Check sheet for the modelled part. Datum: model origin and axes. Units: mm. A direction names the side the tool comes from. Coordinates: 2 decimals unless noted, no trailing zeros. Loops run counter-clockwise (first coordinate to the right, second up) from the corner with the lowest first, then second, coordinate; pieces in that order, holes last.
from build123d import *

# Parameters (mm, degrees)
F1_DEPTH  = 43.5
F2_W      = 170
F2_H      = 80
F3_DEPTH  = 4
F5_DEPTH  = 25
F6_W      = 25
F6_H      = 2
F7_DEPTH  = 43.5
F9_DEPTH  = 25
F10_W     = 25
F10_H     = 0.3
F11_DEPTH = 18.5
F13_DEPTH = 18.5
F14_W     = 25
F14_H     = 0.3
F15_DEPTH = 18.5
F16_W     = 76.6
F16_H     = 2
F17_DEPTH = 25


with BuildPart() as f1:
    # F0 (on Top) → F1 (new body)
    with BuildSketch(Plane.XY):
        Polygon((-166, 0), (-166, 36), (0, 36), (0, 40), (-170, 40), (-170, -40), (0, -40), (0, -36), (-166, -36), align=None)
    extrude(amount=F1_DEPTH)

    # F2 (on face) → F3 (join)
    with BuildSketch(Plane.XY.offset(43.5)):
        with Locations((-85, 0)):
            Rectangle(F2_W, F2_H)
    extrude(amount=F3_DEPTH)

    # F4 (on face) → F5 (cut)
    with BuildSketch(Plane.XY):
        Polygon((0, -36), (-166, -36), (-166, 0), (-166, 36), (0, 36), (0, 38), (-168, 38), (-168, -38), (0, -38), align=None)
    extrude(amount=F5_DEPTH, mode=Mode.SUBTRACT)

    # F6 (on face) → F7 (cut)
    with BuildSketch(Plane.XY):
        with Locations((-12.5, -37)):
            Rectangle(F6_W, F6_H)
        with Locations((-12.5, 37)):
            Rectangle(F6_W, F6_H)
    extrude(amount=F7_DEPTH, mode=Mode.SUBTRACT)

    # F8 (on face) → F9 (cut)
    with BuildSketch(Plane(origin=(0, 0, 0), x_dir=(1, 0, 0), z_dir=(0, 0, -1))):
        Polygon((-168, -38), (-168, 38), (0, 38), (0, 38.3), (-168.3, 38.3), (-168.3, -38.3), (0, -38.3), (0, -38), align=None)
    extrude(amount=-F9_DEPTH, mode=Mode.SUBTRACT)

    # F10 (on face) → F11 (cut)
    with BuildSketch(Plane(origin=(0, 0, 25), x_dir=(1, 0, 0), z_dir=(0, 0, -1))):
        with Locations((-12.5, 38.15)):
            Rectangle(F10_W, F10_H)
    extrude(amount=-F11_DEPTH, mode=Mode.SUBTRACT)

    # F12 (on face) → F13 (cut)
    with BuildSketch(Plane(origin=(0, 0, 25), x_dir=(1, 0, 0), z_dir=(0, 0, -1))):
        Polygon((-166, -36), (-166, 36), (-25, 36), (-25, 36.3), (-166.3, 36.3), (-166.3, -36.3), (-25, -36.3), (-25, -36), align=None)
    extrude(amount=-F13_DEPTH, mode=Mode.SUBTRACT)

    # F14 (on face) → F15 (cut)
    with BuildSketch(Plane(origin=(0, 0, 25), x_dir=(1, 0, 0), z_dir=(0, 0, -1))):
        with Locations((-12.5, -38.15)):
            Rectangle(F14_W, F14_H)
    extrude(amount=-F15_DEPTH, mode=Mode.SUBTRACT)

    # F16 (on face) → F17 (cut)
    with BuildSketch(Plane.YZ):
        with Locations((0, 44.5)):
            Rectangle(F16_W, F16_H)
    extrude(amount=-F17_DEPTH, mode=Mode.SUBTRACT)


solid = f1.part
(1) Set-up check for faces 1 (the face through (-85, 38.3, 12)), 2 (the face through (0, 0, 47)): record each of +Z, -Z, +X, -X, +Y, -Y from which the full face is reachable in a straight line by a thin tool's end or side.
(2) Draft check along Y on faces 3 (the face through (-170, -1, 23)), 4 (the face through (-97, 36.3, 34)), 5 (the face through (-86, 40, 23)). Enter one of: pulls with the +Y half, pulls with the -Y half, needs draft (parallel to the pull), parting line crosses it, or undercut.
(3) Section check D-D, the plane x = -80. Enter the section's corners in (y, z).
(4) Section check B-B, the plane y = -0.5. Enter the section's corners in (x, z).
(5) Gauge pin test, flat ends, axial feed: P1, Ø10, axis at y = 6, z = 31, coming from the +X side; P2, Ø2, axis at y = -22, z = 8, coming from the +X side; P3, Ø1, axis at x = -124.5, y = 9.5, coming from the -Z side. Record the tip position at first contact, or that the pin passes through.
(6) Section check A-A, the plane x = -13. Enter the section's corners in (y, z).
(7) Scan lines: line 1 along Y through (x, z) = (-151, 31.5); line 2 along Y through (x, z) = (-129.5, 7.5); line 3 along Z through (x, y) = (-45, 23.5). Record each from-to range of solid material in increasing order.
(8) Section check C-C, the plane z = 12.5. Enter the section's corners in (x, y).
Determined:
1. face 1: -Z, +X
1. face 2: +Z, -Z, +X, +Y, -Y
2. face 3: needs draft
2. face 4: undercut
2. face 5: pulls with the +Y half
3. outline: (-40, 0) - (-38.3, 0) - (-38.3, 25) - (-36.3, 25) - (-36.3, 43.5) - (36.3, 43.5) - (36.3, 25) - (38.3, 25) - (38.3, 0) - (40, 0) - (40, 47.5) - (-40, 47.5) - close
4. outline: (-170, 0) - (-168.3, 0) - (-168.3, 25) - (-166.3, 25) - (-166.3, 43.5) - (-25, 43.5) - (-25, 45.5) - (0, 45.5) - (0, 47.5) - (-170, 47.5) - close
5. P1: stops at x = -166.3
5. P2: stops at x = -168.3
5. P3: stops at z = 43.5
6. outline: (-40, 0) - (-38.3, 0) - (-38.3, 45.5) - (38.3, 45.5) - (38.3, 0) - (40, 0) - (40, 47.5) - (-40, 47.5) - close
7. line 1: y = -40 to -36.3, 36.3 to 40
7. line 2: y = -40 to -38.3, 38.3 to 40
7. line 3: z = 43.5 to 47.5
8. outline: (-170, -40) - (0, -40) - (0, -38.3) - (-168.3, -38.3) - (-168.3, 38.3) - (0, 38.3) - (0, 40) - (-170, 40) - close
